The listing builds one solid part. Answer for the finished solid, in the listing's coordinates (mm). A direction names the side the tool comes from. Give positions to 0.01 mm unless a question says otherwise; leave off trailing zeros. Order: outer loops, then holes, each group sorted by start corner. A loop starts at its lowest first (then second) coordinate and runs counter-clockwise, first axis right, second up. Notation, with made-up numbers: (35.5, 44.5) -> (88.5, 44.5) arc R25 ccw to (88.5, 67.5) -> close; hole circle Ø11 at (-21.5, 86). An arc over 180 degrees is marked (long way). Write item = value, one per line. Start each with the question number.
```python
from build123d import *

# Parameters (mm, degrees)
SKETCH_1_W                   = 66
SKETCH_1_H                   = 30
EXTRUDE_1_DEPTH              = 12
SKETCH_2_R                   = 23
CUT_EXTRUDE_1_DEPTH          = 74.484692283
HOLE_WIZARD_M4_1_D           = 4.8
HOLE_WIZARD_M4_1_CBORE_D     = 8
HOLE_WIZARD_M4_1_CBORE_DEPTH = 4


with BuildPart() as part:
    # 草图1 → 凸台-拉伸1 (new body)
    with BuildSketch(Plane.XY):
        with Locations((33, 15)):
            Rectangle(SKETCH_1_W, SKETCH_1_H)
    extrude(amount=EXTRUDE_1_DEPTH)

    # 草图2 → 切除-拉伸1 (cut, through all)
    with BuildSketch(Plane.XY.offset(12)):
        with Locations((33, 30.1)):
            Circle(SKETCH_2_R)
    extrude(amount=-CUT_EXTRUDE_1_DEPTH, mode=Mode.SUBTRACT)

    # M4 六角凹头螺钉的柱形沉头孔1 (through all)
    with Locations(Plane.XZ):
        with Locations((61, 6), (5, 6)):
            CounterBoreHole(HOLE_WIZARD_M4_1_D / 2, HOLE_WIZARD_M4_1_CBORE_D / 2, HOLE_WIZARD_M4_1_CBORE_DEPTH)


solid = part.part
```
Item 1: Flat-ended cylindrical pins translate along their axes: pin 1 (4.5 mm diameter, centred on x = 5, z = 6, fed in from +Y); pin 2 (2.5 mm diameter, centred on x = 3.5, z = 7, fed in from -Y); pin 3 (3 mm diameter, centred on x = 47.5, z = 8.5, fed in from +Y). Find the tip coordinate at first contact, or state that the pin passes through.
Item 2: A cutting plane is placed at D-D, the plane y = 15.5. Write down the section's boundary in (x, z).
Item 3: A cutting plane is placed at C-C, the plane z = 6. Write down the section's boundary in (x, y).
Item 4: Consider L1, parallel to X at y = 2, z = 5.75; L2, parallel to Z at x = 61, y = 11; L3, parallel to Z at x = 61, y = 2. Determine where each line is inside the solid, lowest interval first. Write a range as from..to.
Item 5: A cutting plane is placed at B-B, the plane x = 61. Write down the section's boundary in (y, z).
Item 6: A cutting plane is placed at A-A, the plane y = 25. Write down the section's boundary in (x, z).
Item 7: Which of the six approach directions +Z, -Z, +X, -X, +Y, -Y give full straight-line access (tool end or side, diameter ignored) to faces 1 (the flat face through (33, 5, 12)), 2 (the flat face through (7, 4, 4))?
Item 8: The mould has two halves that part along Z. Classify faces 3 (the flat face through (33, 5, 0)), 4 (the cylindrical face through (64.695, 1.972, 4.468)), 5 (the flat face through (66, 15, 6)): +Z half, -Z half, draft (parallel to the pull), parting line (faces both ways), or undercut.
Check values:
q1.pin_1 = through
q1.pin_2 = 4
q1.pin_3 = 13.58
q2.outline = (0, 0) -> (15.23, 0) -> (15.23, 12) -> (0, 12) -> close; (50.77, 0) -> (66, 0) -> (66, 12) -> (50.77, 12) -> close; hole circle Ø4.8 at (5, 6); hole circle Ø4.8 at (61, 6)
q3.outline = (0, 0) -> (1, 0) -> (1, 4) -> (2.6, 4) -> (2.6, 30) -> (0, 30) -> close; (7.4, 4) -> (9, 4) -> (9, 0) -> (57, 0) -> (57, 4) -> (58.6, 4) -> (58.6, 30) -> (56, 30) arc R23 cw to (10, 30) -> (7.4, 30) -> close; (63.4, 4) -> (65, 4) -> (65, 0) -> (66, 0) -> (66, 30) -> (63.4, 30) -> close
q4.L1 = 0..1.01, 8.99..57.01, 64.99..66
q4.L2 = 0..3.6, 8.4..12
q4.L3 = 0..2, 10..12
q5.outline = (0, 0) -> (30, 0) -> (30, 3.6) -> (4, 3.6) -> (4, 2) -> (0, 2) -> close; (0, 10) -> (4, 10) -> (4, 8.4) -> (30, 8.4) -> (30, 12) -> (0, 12) -> close
q6.outline = (0, 0) -> (10.57, 0) -> (10.57, 12) -> (0, 12) -> close; (55.43, 0) -> (66, 0) -> (66, 12) -> (55.43, 12) -> close; hole circle Ø4.8 at (5, 6); hole circle Ø4.8 at (61, 6)
q7.face_1 = +Z, +X, -X, +Y, -Y
q7.face_2 = -Y
q8.face_3 = -Z half
q8.face_4 = undercut
q8.face_5 = draft
